```python
from build123d import *

# Parameters (mm, degrees)
SKETCH1_R                       = 3
BOSS_EXTRUDE1_DEPTH             = 30
SKETCH2_R                       = 6.099567635
BOSS_EXTRUDE2_DEPTH             = 10
CUT_EXTRUDE1_DEPTH              = 41.919548515
CUT_EXTRUDE1_DEPTH_BACK         = 41.919548515
SKETCH3_W                       = 2.43383409
SKETCH3_H                       = 2.25
SKETCH3_W_2                     = 2.704181163
TAP_DRILL_FOR_M3X0_5_TAP1_D     = 2.5
TAP_DRILL_FOR_M3X0_5_TAP1_DEPTH = 2.999994
TAP_DRILL_FOR_M3X0_5_TAP1_TIP   = 0.751075774


with BuildPart() as part:
    # Sketch1 → Boss-Extrude1 (new body)
    with BuildSketch(Plane.XY):
        Circle(SKETCH1_R)
    extrude(amount=BOSS_EXTRUDE1_DEPTH)

    # Sketch2 → Boss-Extrude2 (add)
    with BuildSketch(Plane.XY.offset(30)):
        Circle(SKETCH2_R)
    extrude(amount=BOSS_EXTRUDE2_DEPTH)

    # Sketch3 → Cut-Extrude1 (cut, two sides: drawn at the far end of the back side and taken through both)
    with BuildSketch(Plane(origin=(0, 0, 0), x_dir=(1, 0, 0), z_dir=(0, 1, 0)).offset(-CUT_EXTRUDE1_DEPTH_BACK)):
        with Locations((3.716917045, -1.125)):
            Rectangle(SKETCH3_W, SKETCH3_H)
        with Locations((-3.852090582, -1.125)):
            Rectangle(SKETCH3_W_2, SKETCH3_H)
    extrude(amount=CUT_EXTRUDE1_DEPTH + CUT_EXTRUDE1_DEPTH_BACK, mode=Mode.SUBTRACT)

    # Tap Drill for M3x0.5 Tap1
    with Locations(Plane(origin=(0, 0, 0), x_dir=(-1, 0, 0), z_dir=(0, 0, -1))):
        with Locations((0, 0)):
            Hole(TAP_DRILL_FOR_M3X0_5_TAP1_D / 2, depth=TAP_DRILL_FOR_M3X0_5_TAP1_DEPTH)
            with Locations((0, 0, -(TAP_DRILL_FOR_M3X0_5_TAP1_DEPTH + TAP_DRILL_FOR_M3X0_5_TAP1_TIP / 2))):  # 118° drill point
                Cone(0, TAP_DRILL_FOR_M3X0_5_TAP1_D / 2, TAP_DRILL_FOR_M3X0_5_TAP1_TIP, mode=Mode.SUBTRACT)


solid = part.part
```
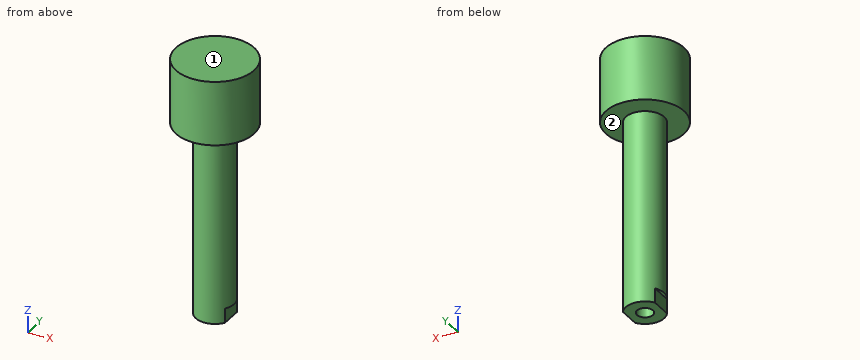
Could you check a few things on this model? Use its own coordinates, in mm. Face numbers are marked on the shaded views. A direction names the side the tool comes from. Coordinates: 2 decimals unless noted, no trailing zeros. Write each loop counter-clockwise with the first axis right and the second up, starting at its lowest first coordinate (ties: lowest second). Pieces come first, ordered by that corner, then holes. Notation, with made-up numbers: (29, 16) -> (83, 16) arc R27 cw to (83, 47) -> close; hole circle Ø8 at (6.5, 46.25). An arc over 180 degrees is marked (long way). Write item = value, one per line. Start each with the question number.
(1) Which directions (+Z, -Z, +X, -X, +Y, -Y) give clear straight access to the entire face, cutting with the end or side of a thin tool? Please do the marked faces 1 and 2.
(2) Will these pins go through, and if not, where does the flat tip stop? pin 1 (1.1 mm diameter, centred on y = 0, z = 1, fed in from +X); pin 2 (6 mm diameter, centred on x = -2.5, y = 2, fed in from -Z); pin 3 (1 mm diameter, centred on y = 0, z = 12.5, fed in from -X); pin 4 (4 mm diameter, centred on y = -4.5, z = 31, fed in from +X).
(3) I need wall thicknesses on line 1 (Y direction, x = 0, z = 2.2); line 2 (X direction, y = 0, z = 1.45); line 3 (Z direction, x = 3, y = 2.5). Which ranges of each line are inside material? Lowest first, please. Write a range as [from, to].
(4) I want a section at B-B (x = -4). Please give me the cut outline in (y, z).
(5) I want a section at D-D (z = 38.5). Please give me the cut outline in (x, y).
(6) I want a section at A-A (z = 29). Please give me the cut outline in (x, y), plus the area to 3 significant figures.
(7) I want a section at C-C (y = 5). Please give me the cut outline in (x, z), plus the area to 3 significant figures.
Result set:
q1.face_1 = +Z, +X, -X, +Y, -Y
q1.face_2 = -Z
q2.pin_1 = 2.5
q2.pin_2 = 0
q2.pin_3 = -3
q2.pin_4 = 5.56
q3.line_1 = [-3, -1.25], [1.25, 3]
q3.line_2 = [-2.5, -1.25], [1.25, 2.5]
q3.line_3 = [30, 40]
q4.outline = (-4.6, 30) -> (4.6, 30) -> (4.6, 40) -> (-4.6, 40) -> close
q5.outline = circle Ø12.2 at (0, 0)
q6.outline = circle Ø6 at (0, 0)
q6.area = 28.3 mm2
q7.outline = (-3.49, 30) -> (3.49, 30) -> (3.49, 40) -> (-3.49, 40) -> close
q7.area = 69.9 mm2
